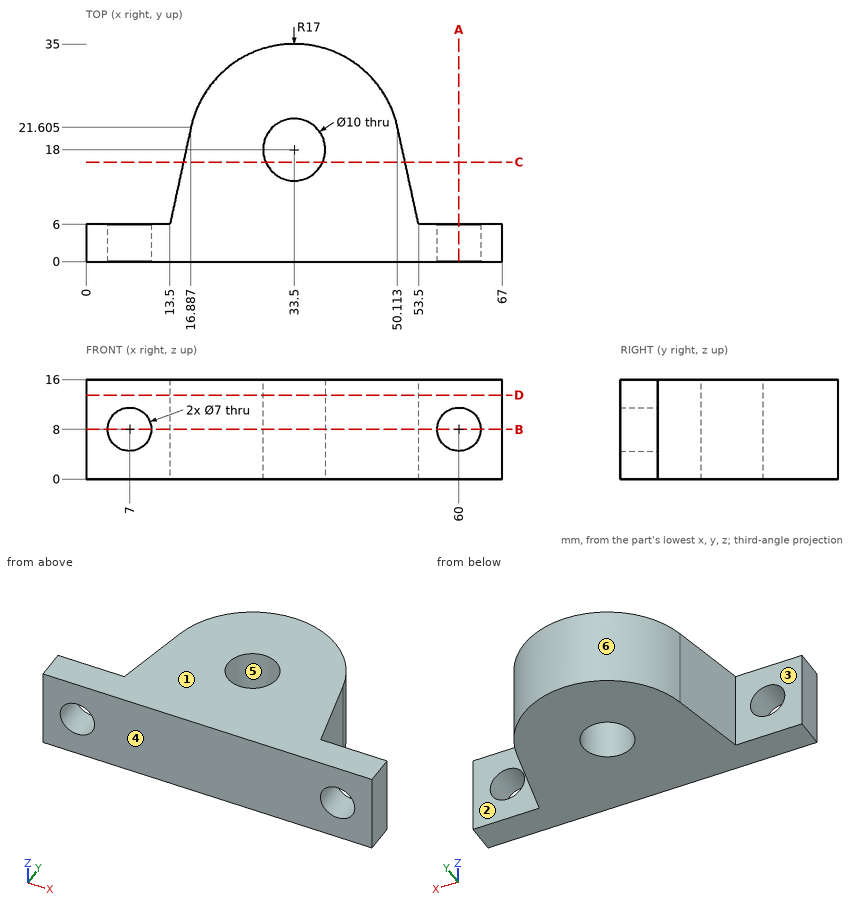
For this review, use the dimensioned drawing (mm, ordinates from the lowest corner) and the shaded views. A direction names the side the tool comes from. Round coordinates to 2 decimals unless told otherwise and drop trailing zeros. Order: outer loops, then holes, each group sorted by start corner. A loop starts at its lowest first (then second) coordinate and runs counter-clockwise, first axis right, second up. Notation, with made-up numbers: (77, 70.5) - (132, 70.5) arc R28 ccw to (132, 88.5) - close; hole circle Ø2 at (-17.5, 50.5). An arc over 180 degrees is marked (long way). Use one line per item in the form item = value.
Q1. Add section B-B on z = 8. Give the boundary of the cut face in (x, y) (1 decimal), then the cut area to 3 significant figures.
Response values:
outline = (0, 0) - (3.5, 0) - (3.5, 6) - (0, 6) - close; (10.5, 0) - (56.5, 0) - (56.5, 6) - (53.5, 6) - (50.1, 21.6) arc R17 ccw to (16.9, 21.6) - (13.5, 6) - (10.5, 6) - close; (63.5, 0) - (67, 0) - (67, 6) - (63.5, 6) - close; hole circle Ø10 at (33.5, 18)
area = 1,140 mm^2
Q2. Add section C-C on y = 16. Give the boundary of the cut face in (x, z), then the cut area to 3 significant figures.
Response values:
outline = (15.67, 0) - (28.92, 0) - (28.92, 16) - (15.67, 16) - close; (38.08, 0) - (51.33, 0) - (51.33, 16) - (38.08, 16) - close
area = 424 mm^2
Q3. To check wall thickness, follow line 1 (X direction, y = 4.3, z = 8); line 2 (Z direction, x = 60, y = 3.85); line 3 (Y direction, x = 33.5, z = 9). State the ranges of each line that lie inside material, in increasing order.
Response values:
line_1 = 0 to 3.5, 10.5 to 56.5, 63.5 to 67
line_2 = 0 to 4.5, 11.5 to 16
line_3 = 0 to 13, 23 to 35
Q4. Add section A-A on x = 60. Give the boundary of the cut face in (y, z), then the cut area to 3 significant figures.
Response values:
outline = (0, 0) - (6, 0) - (6, 4.5) - (0, 4.5) - close; (0, 11.5) - (6, 11.5) - (6, 16) - (0, 16) - close
area = 54.0 mm^2
Q5. Clearance check with flat-ended pins moving along their axes: P1, Ø3, axis at x = 17.5, z = 14.5, coming from the +Y side (1 decimal); P2, Ø8, axis at x = 60, z = 8, coming from the +Y side; P3, Ø1, axis at y = 20.5, z = 9.5, coming from the +X side. State where each tip first meets the part, or that it passes through.
Response values:
P1 = 26.9
P2 = 6
P3 = 50.46
Q6. Mouldability with a two-part tool opening along X and no side actions: class the marked faces 4, 5 and 6 as pulls with the +X half, pulls with the -X half, needs draft (parallel to the pull), parting line crosses it, or undercut.
Response values:
face_4 = needs draft
face_5 = undercut
face_6 = parting line crosses it
Q7. Tool access review of the marked faces 1, 2 and 3: name each direction out of +Z, -Z, +X, -X, +Y, -Y from which nothing blocks a thin tool from reaching the whole face with its end or side.
Response values:
face_1 = +Z, +X, -X, +Y, -Y
face_2 = +Z, -Z, +X, +Y
face_3 = +Z, -Z, -X, +Y
Q8. Add section D-D on z = 13.5. Give the boundary of the cut face in (x, y) (1 decimal), then the cut area to 3 significant figures.
Response values:
outline = (0, 0) - (67, 0) - (67, 6) - (53.5, 6) - (50.1, 21.6) arc R17 ccw to (16.9, 21.6) - (13.5, 6) - (0, 6) - close; hole circle Ø10 at (33.5, 18)
area = 1,230 mm^2
